Could you check a few things on this model? Use its own coordinates, in mm. A direction names the side the tool comes from. Round coordinates to 2 decimals unless told otherwise and drop trailing zeros. Order: outer loops, then holes, each group sorted by start corner. A loop starts at its lowest first (then second) coordinate and runs counter-clockwise, first axis right, second up. Notation, with made-up numbers: (-13, 0) -> (25, 0) arc R16 cw to (25, 28) -> close; hole circle Ø10 at (50.5, 67.5). An arc over 180 degrees is marked (long way). One line per question, with ' | ' between items.
```python
from build123d import *

# Parameters (mm, degrees)
SKETCH_1_R      = 1
EXTRUDE_1_DEPTH = 15
EXTRUDE_2_DEPTH = 1.5
SKETCH_3_R      = 1
EXTRUDE_3_DEPTH = 3
SKETCH_4_W      = 3
SKETCH_4_H      = 2
EXTRUDE_4_DEPTH = 2.3
EXTRUDE_5_DEPTH = 7
EXTRUDE_6_DEPTH = 7
FILLET_1_R      = 1
FILLET_2_R      = 1
FILLET_3_R      = 2
CHAMFER_2_SIZE  = 2


# Some blends are built 0.0001 mm under size
with BuildPart() as part:
    # Эскиз1 → Бобышка-Вытянуть1 (new body)
    with BuildSketch(Plane.XY):
        Circle(SKETCH_1_R)
    extrude(amount=EXTRUDE_1_DEPTH)

    # Эскиз2 → Бобышка-Вытянуть2 (add)
    with BuildSketch(Plane(origin=(0, 0, 1.5), x_dir=(-1, 0, 0), z_dir=(0, 0, -1))):
        with BuildLine():
            Line((0, 1.201036303), (7.6, 1.201036303))
            ThreePointArc((7.6, 1.201036303), (8.8, 0.001036303), (7.6, -1.198963697))
            Line((7.6, -1.198963697), (0, -1.198963697))
            ThreePointArc((0, -1.198963697), (-1.2, 0.001036303), (0, 1.201036303))
        make_face()
    extrude(amount=-EXTRUDE_2_DEPTH)

    # Эскиз3 → Бобышка-Вытянуть3 (add)
    with BuildSketch(Plane.XY.offset(3)):
        with Locations((-7.6, 0.001036303)):
            Circle(SKETCH_3_R)
    extrude(amount=-EXTRUDE_3_DEPTH)

    # Эскиз4 → Бобышка-Вытянуть4 (add)
    with BuildSketch(Plane.XY.offset(3)):
        with Locations((-1.5, 0)):
            Rectangle(SKETCH_4_W, SKETCH_4_H)
    extrude(amount=EXTRUDE_4_DEPTH)

    # Эскиз5 → Бобышка-Вытянуть5 (add)
    with BuildSketch(Plane(origin=(0, 0, 4), x_dir=(-1, 0, 0), z_dir=(0, 0, -1))):
        Polygon((0, 0), (-0.782172325, -4.938441703), (-5.720614028, -4.156269378), (-4.938441703, 0.782172325), align=None)
    extrude(amount=-EXTRUDE_5_DEPTH)

    # Эскиз6 → Бобышка-Вытянуть6 (add)
    with BuildSketch(Plane(origin=(0, 0, 4), x_dir=(-1, 0, 0), z_dir=(0, 0, -1))):
        with BuildLine():
            Line((-0.987688341, 0.156434465), (-4.938441703, 0.782172325))
            add(Edge.make_bspline(
                [(-4.938441703, 0.782172325), (-6.035924713, -6.147062691), (-16.447307855, -8.707880394), (-20.782172325, -6.582481038)],
                knots=[0, 0, 0, 0, 1, 1, 1, 1], degree=3))
            add(Edge.make_bspline(
                [(-20.782172325, -6.582481038), (-19.502585952, -9.761328662), (-5.677351674, -8.787425093), (-2.826630593, -4.614631324)],
                knots=[0, 0, 0, 0, 1, 1, 1, 1], degree=3))
            Line((-2.826630593, -4.614631324), (-0.782172325, -4.938441703))
            Line((-0.782172325, -4.938441703), (-0.156434465, -0.987688341))
            ThreePointArc((-0.156434465, -0.987688341), (-0.809016994, -0.587785252), (-0.987688341, 0.156434465))
        make_face()
    extrude(amount=-EXTRUDE_6_DEPTH)

    # Скругление1
    fillet_1_edges = [part.edges().sort_by_distance(p)[0] for p in [
        (4.938441703, 0.782172325, 7.5),
    ]]
    fillet(fillet_1_edges, radius=FILLET_1_R)

    # Скругление2
    # the kernel refuses this fillet: 1 mm, written as the material it adds along each edge
    with BuildSketch(Plane(origin=(0.156434465, -0.987688341, 11), x_dir=(-0.9945218953682737, 0.10452846326764978, 0), z_dir=(0, 0, -1))) as fillet_2_piece_1:
        with BuildLine():
            CenterArc((0.776457135, -0.965925826), FILLET_2_R, 105, 60)
            Line((-0.189468691, -0.707106781), (-0.208787208, -0.7019304))
            Line((-0.208787208, -0.7019304), (-0.019318517, 0.005176381))
            Line((-0.019318517, 0.005176381), (0.005176381, 0.019318517))
            ThreePointArc((0.005176381, 0.019318517), (0.258819045, -0.014074174), (0.512461709, 0.019318517))
            Line((0.512461709, 0.019318517), (0.51763809, 0))
        make_face()
    extrude(amount=7)

    # Скругление3
    fillet_3_edges = [part.edges().sort_by_distance(p)[0] for p in [
        (0.987688341, 0.156434465, 7.5),
    ]]
    fillet(fillet_3_edges, radius=FILLET_3_R)

    # Фаска2
    chamfer_2_edges = [part.edges().sort_by_distance(p)[0] for p in [
        (-3, 0, 5.3),
    ]]
    chamfer(chamfer_2_edges, length=CHAMFER_2_SIZE - 0.0001)  # a hair under: the kernel refuses the full size


solid = part.part
```
1. I need wall thicknesses on probe 1 along Z at (x, y) = (0.75, -1.75); probe 2 along Z at (x, y) = (-7.5, 0); probe 3 along X at (y, z) = (-0.75, 12.75). Which ranges of each line are inside material? Lowest first, please.
From the geometry:
probe 1: z = 4 to 11 | probe 2: z = 0 to 3 | probe 3: x = -0.66 to 0.66
2. If we mould it in two halves opening along X, with no side actions, what happens to faces 1 (the face through (-8.8, 0, 2.2)), 2 (the face through (-4, -1.199, 2)), 3 (the face through (1.36, 0.4, 7.45))? For each: pulls with the +X half, pulls with the -X half, needs draft (parallel to the pull), parting line crosses it, or undercut.
From the geometry:
face 1: pulls with the -X half | face 2: needs draft | face 3: undercut
3. I'm going to push flat-ended pins straight in: pin 1 (2.5 mm diameter, centred on x = -1.5, z = 4.5, fed in from +Y); pin 2 (2.5 mm diameter, centred on x = -3.5, y = -0.5, fed in from -Z); pin 3 (4.5 mm diameter, centred on x = 12.5, y = -3, fed in from -Z); pin 4 (1.8 mm diameter, centred on x = -2, z = 3.5, fed in from -Y). Where does each tip first touch, or does it pass through?
From the geometry:
pin 1: stops at y = 1 | pin 2: stops at z = 1.5 | pin 3: passes through | pin 4: stops at y = -1.2
4. On a 3-axis mill with a long thin cutter (end or side, diameter ignored), from which of +Z, -Z, +X, -X, +Y, -Y can I reach the whole of each face in a straight line? I mean faces 4 (the face through (-8.6, 0, 0.8)), 5 (the face through (1.79, -4.78, 7.45)), 6 (the face through (3.122, 0.494, 7.451)), 7 (the face through (1.2, 0, 2.2)). Say none if no direction works.
From the geometry:
face 4: -Z | face 5: +Z, -Z, -Y | face 6: +Z, -Z, +Y | face 7: -Z, +X
5. I want a section at A-A on z = 13. List the corners of the cut face in (x, y) for me, and give its area (3 significant figures).
From the geometry:
outline: circle Ø2 at (0, 0) | area: 3.14 mm²
